For this review, take the finished solid that the model builds, in its own axes (mm). A direction names the side the tool comes from. Coordinates: 2 decimals unless noted, no trailing zeros. Write each loop counter-clockwise with the first axis right and the second up, starting at its lowest first coordinate (ties: lowest second). Pieces come first, ordered by that corner, then holes. Notation, with made-up numbers: (-18.75, -31.75) -> (-3.75, -31.75) arc R20 ccw to (-3.75, -4.75) -> close; hole circle Ø2 at (-31, -9). An arc over 180 degrees is marked (long way). One line per item, written item: value. Start each with the question number.
1) For probe 1 along Y at (x, z) = (-19.05, 11.85); probe 2 along X at (y, z) = (-12.25, -0.25); probe 3 along Z at (x, y) = (0, -5.5) (3 decimals), list the stretches that pass through material, from the lowest coordinate up. Write a range as from..to.
2) Mouldability with a two-part tool opening along Z and no side actions: class faces 3 (the cylindrical face through (-0.98, -11.77, 7.43)), 4 (the flat face through (-11.493, -12, 5)), 5 (the flat face through (-19, -12, 9.525)) as released by +Z, released by -Z, zero draft, split by the parting line, or undercut.
3) Add section D-D (y = -1.25). State the section outline as (x, z) points (3 decimals), and give its area (3 significant figures).
4) Add section C-C (x = 19.05). State the section outline as (y, z) points (3 decimals), and give its area (3 significant figures).
5) Add section B-B (x = 0). State the section outline as (y, z) points (3 decimals), and give its area (3 significant figures).
6) Add section A-A (y = -6.35). State the section outline as (x, z) points (3 decimals).
7) For pin 1 Ø4 at (x, y) = (-19.05, -17.526) entering from +Z; pin 2 Ø10 at (y, z) = (-12.5, -7.5) entering from +X; pin 3 Ø5 at (y, z) = (-17.5, -4.5) entering from -X; pin 4 Ø7.5 at (y, z) = (-12, 3.5) entering from -X, all flat-tipped, find the tip position at first contact; note any pin that passes through.
8) Machinability: for faces 1 (the cylindrical face through (-0.25, -11.77, -11.49)), 2 (the flat face through (11.493, -12, 5)), which of the approach directions +Z, -Z, +X, -X, +Y, -Y give a long, thin tool a straight path to every point of the face, cutting with its end or side? Answer none if there is none.
from build123d import *

# Parameters (mm, degrees)
F0_R     = 7.493
F1_DEPTH = 23.876
F2_R     = 2.4
F3_DEPTH = 6


with BuildPart() as f1:
    # F0 (on Front) → F1 (new body)
    with BuildSketch(Plane.XZ):
        with BuildLine():
            Line((25.4, 15.525), (-25.4, 15.525))
            Line((-25.4, 15.525), (-25.4, 9.525))
            Line((-25.4, 9.525), (-11.493, 9.525))
            Line((-11.493, 9.525), (-11.493, 0))
            ThreePointArc((-11.493, 0), (0, -11.493), (11.493, 0))
            Line((11.493, 0), (11.493, 9.525))
            Line((11.493, 9.525), (25.4, 9.525))
            Line((25.4, 9.525), (25.4, 15.525))
        make_face()
        Circle(F0_R, mode=Mode.SUBTRACT)
    extrude(amount=F1_DEPTH)

    # F2 (on face) → F3 (cut, through all)
    with BuildSketch(Plane.XY.offset(15.525)):
        with Locations((-19.05, -6.35)):
            Circle(F2_R)
        with Locations((-19.05, -17.526)):
            Circle(F2_R)
        with Locations((19.05, -17.526)):
            Circle(F2_R)
        with Locations((19.05, -6.35)):
            Circle(F2_R)
    extrude(amount=-F3_DEPTH, mode=Mode.SUBTRACT)


solid = f1.part
Numbers:
1. probe 1: -23.88..-19.93, -15.13..-8.75, -3.95..0
1. probe 2: -11.49..-7.49, 7.49..11.49
1. probe 3: -11.493..-7.493, 7.493..15.525
2. face 3: undercut
2. face 4: zero draft
2. face 5: released by -Z
3. outline: (-25.4, 9.525) -> (-11.493, 9.525) -> (-11.493, 0) arc R11.493 ccw to (11.493, 0) -> (11.493, 9.525) -> (25.4, 9.525) -> (25.4, 15.525) -> (-25.4, 15.525) -> close; hole circle Ø14.986 at (0, 0)
3. area: 555 mm²
4. outline: (-23.876, 9.525) -> (-19.926, 9.525) -> (-19.926, 15.525) -> (-23.876, 15.525) -> close; (-15.126, 9.525) -> (-8.75, 9.525) -> (-8.75, 15.525) -> (-15.126, 15.525) -> close; (-3.95, 9.525) -> (0, 9.525) -> (0, 15.525) -> (-3.95, 15.525) -> close
4. area: 85.7 mm²
5. outline: (-23.876, -11.493) -> (0, -11.493) -> (0, -7.493) -> (-23.876, -7.493) -> close; (-23.876, 7.493) -> (0, 7.493) -> (0, 15.525) -> (-23.876, 15.525) -> close
5. area: 287 mm²
6. outline: (-25.4, 9.525) -> (-21.45, 9.525) -> (-21.45, 15.525) -> (-25.4, 15.525) -> close; (-16.65, 9.525) -> (-11.493, 9.525) -> (-11.493, 0) arc R11.493 ccw to (11.493, 0) -> (11.493, 9.525) -> (16.65, 9.525) -> (16.65, 15.525) -> (-16.65, 15.525) -> close; (21.45, 9.525) -> (25.4, 9.525) -> (25.4, 15.525) -> (21.45, 15.525) -> close; hole circle Ø14.986 at (0, 0)
7. pin 1: through
7. pin 2: x = 11.22
7. pin 3: x = -11.32
7. pin 4: x = -11.49
8. face 1: -Z, +Y, -Y
8. face 2: -Z, +X, +Y, -Y
